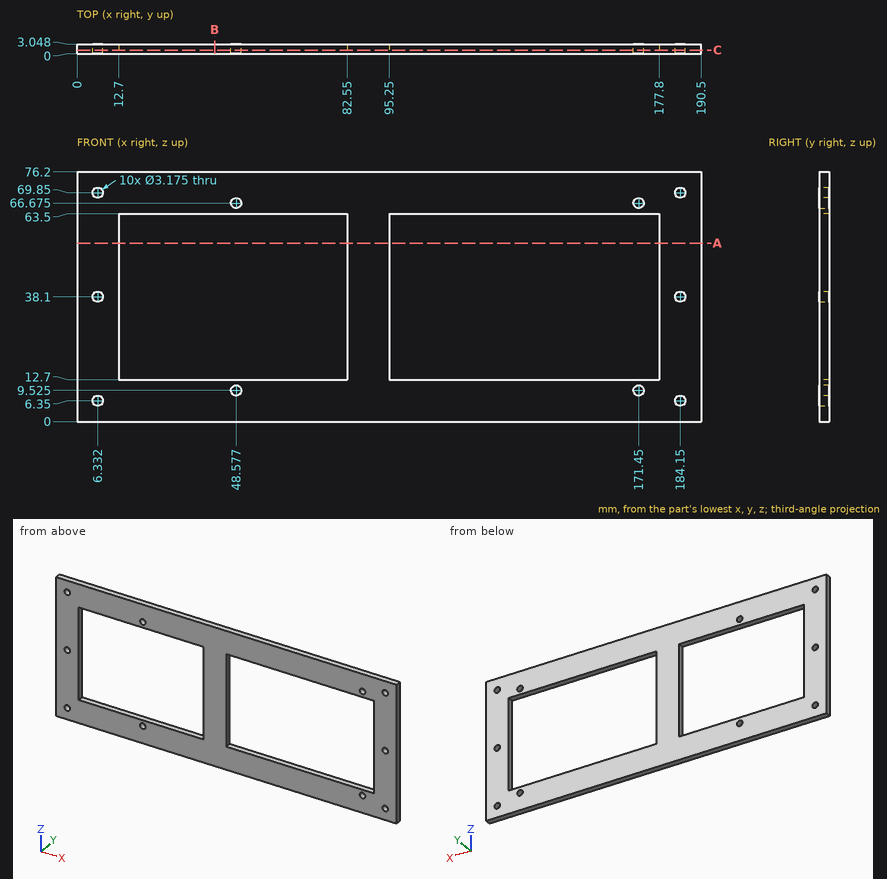
Geometry: see drawing. Coordinates: mm, zero at the bounding-box minimum. Give positions to 0.01 mm unless a question says otherwise; leave off trailing zeros. Loops run counter-clockwise (first coordinate to the right, second up) from the corner with the lowest first, then second, coordinate; pieces in that order, holes last. Notation, with made-up numbers: M 51.25,39.5 L 110.25,39.5 A27 ccw 110.25,57.5 Z; hole C -30.75,86 d1. An arc over 180 degrees is marked long. Use one line per item in the form item = value.
1. Section query B-B, the plane x = 42. Return the cut outline in (y, z).
Numbers:
outline = M 0,0 L 3.05,0 L 3.05,12.7 L 0,12.7 Z; M 0,63.5 L 3.05,63.5 L 3.05,76.2 L 0,76.2 Z
2. Section query A-A, the plane z = 54.5. Return the cut outline in (x, y), and give its area (3 significant figures).
Numbers:
outline = M 0,0 L 12.7,0 L 12.7,3.05 L 0,3.05 Z; M 82.55,0 L 95.25,0 L 95.25,3.05 L 82.55,3.05 Z; M 177.8,0 L 190.5,0 L 190.5,3.05 L 177.8,3.05 Z
area = 116 mm²
3. Line query: L1, parallel to X at y = 1.9, z = 13.5; L2, parallel to Z at x = 171.45, y = 2.1; L3, parallel to Z at x = 32.5, y = 0.25. Output: solid intervals per line, ascending.
Numbers:
L1 = 0 to 12.7, 82.55 to 95.25, 177.8 to 190.5
L2 = 0 to 7.94, 11.11 to 12.7, 63.5 to 65.09, 68.26 to 76.2
L3 = 0 to 12.7, 63.5 to 76.2
4. Section query C-C, the plane y = 1.2. Count the separate pieces of the cut face and the enclosed holes in it.
Numbers:
separate_pieces = 1
enclosed_holes = 12
